For this review, take the finished solid that the model builds, in its own axes (mm). A direction names the side the tool comes from. Round coordinates to 2 decimals unless told otherwise and drop trailing zeros. Loops run counter-clockwise (first coordinate to the right, second up) from the corner with the lowest first, then second, coordinate; pieces in that order, holes last.
1) Take a section at C-C (y = 0). State the section outline as (x, z) points, then the cut area to 3 significant figures.
2) Tool access review of faces 1 (the flat face through (12, -17.828, -27)), 2 (the flat face through (12, -32.828, -19)), 3 (the cylindrical face through (12.325, -39.352, -60.393)): name each direction out of +Z, -Z, +X, -X, +Y, -Y from which nothing blocks a thin tool from reaching the whole face with its end or side.
3) Mouldability with a two-part tool opening along Z and no side actions: class faces 4 (the flat face through (0, 11.3, -26)), 5 (the cylindrical face through (12.32, -22.07, 24.3)), 6 (the flat face through (12.325, 18.802, -57.745)) as pulls with the +Z half, pulls with the -Z half, needs draft (parallel to the pull), parting line crosses it, or undercut.
4) Wall thickness on L1, parallel to Y at x = 11.5, z = -9.5; L2, parallel to Z at x = 7.5, y = 11.5; L3, parallel to Z at x = 7, y = 16: over which ranges is each line inside the solid? List them lowest first.
5) Insertion check: pin 1 (7.5 mm diameter, centred on x = 17, z = -40, fed in from -Y); pin 2 (10 mm diameter, centred on x = 17, y = 22.5, fed in from +Z); pin 3 (8 mm diameter, centred on x = 5, y = 3.5, fed in from +Z); pin 4 (10 mm diameter, centred on y = 5, z = -37, fed in from -X). Each pin has a flat end and moves straight along its axis. Give the tip position at first contact, or say it passes through.
6) Take a section at B-B (x = 18.5). State the section outline as (y, z) points, then the cut area to 3 significant figures.
7) Take a section at D-D (z = -32). State the section outline as (x, y) points.
8) Take a section at A-A (z = 6.5). State the section outline as (x, y) points.
```python
from build123d import *

# Parameters (mm, degrees)
F1_DEPTH = 25


# Not quite as in the source:
# - a feature names something its author has since deleted; it is built from what else it names


with BuildPart() as f1:
    # F0 (on Right) → F1 (new body)
    with BuildSketch(Plane.YZ):
        with BuildLine():
            Line((21.3200338185, 0), (17.8281293297, 0))
            ThreePointArc((17.8281293297, 0), (16.0680734174, -7.7239376), (11.135423556, -13.9228063846))
            Line((11.135423556, -13.9228063846), (11.135423556, -30.8818460833))
            ThreePointArc((11.135423556, -30.8818460833), (16.4953904054, -28.3828851715), (21.3200338185, -24.9628170138))
            Line((21.3200338185, -24.9628170138), (21.3200338185, 0))
        make_face()
        with BuildLine():
            ThreePointArc((-17.8281293297, 0), (0, 17.8281293297), (17.8281293297, 0))
            Line((17.8281293297, 0), (21.3200338185, 0))
            Line((21.3200338185, 0), (21.3200338185, -24.9628170138))
            ThreePointArc((21.3200338185, -24.9628170138), (29.8126055788, -13.7438940584), (32.8281293297, 0))
            ThreePointArc((32.8281293297, 0), (32.5773816899, 4.0497256101), (31.8289692891, 8.0375860357))
            Line((31.8289692891, 8.0375860357), (31.3856816717, 9.6241914615))
            ThreePointArc((31.3856816717, 9.6241914615), (28.3999929291, 16.4659186477), (23.9458348633, 22.4562478608))
            ThreePointArc((23.9458348633, 22.4562478608), (8.5005350475, 17.8111454186), (2.3973170077, 32.7404787144))
            ThreePointArc((2.3973170077, 32.7404787144), (-22.3493472221, 24.0456389815), (-32.8281293297, 0))
            Line((-32.8281293297, 0), (-17.8281293297, 0))
        make_face()
        with BuildLine():
            Line((-17.8281293297, -27.5652658229), (-17.8281293297, 0))
            Line((-17.8281293297, 0), (-32.8281293297, 0))
            ThreePointArc((-32.8281293297, 0), (-28.8353100436, -15.6911111771), (-17.8281293297, -27.5652658229))
        make_face()
        with BuildLine():
            Line((-17.8281293297, -49.2888468657), (-17.8281293297, -27.5652658229))
            ThreePointArc((-17.8281293297, -27.5652658229), (-28.8353100436, -15.6911111771), (-32.8281293297, 0))
            Line((-32.8281293297, 0), (-32.8281293297, -39.2883635356))
            ThreePointArc((-32.8281293297, -39.2883635356), (-23.2296585262, -41.1410511261), (-17.8281293297, -49.2888468657))
        make_face()
        with BuildLine():
            ThreePointArc((21.3200338185, -24.9628170138), (16.4953904054, -28.3828851715), (11.135423556, -30.8818460833))
            Line((11.135423556, -30.8818460833), (11.135423556, -91.2536308169))
            Line((11.135423556, -91.2536308169), (16.2277286872, -91.2536308169))
            Line((16.2277286872, -91.2536308169), (16.3531204545, -89.621300844))
            Line((16.3531204545, -89.621300844), (21.3200338185, -24.9628170138))
        make_face()
        with BuildLine():
            Line((-17.8281293297, -49.3592731655), (-17.8281293297, -49.2888468657))
            ThreePointArc((-17.8281293297, -49.2888468657), (-23.2296585262, -41.1410511261), (-32.8281293297, -39.2883635356))
            Line((-32.8281293297, -39.2883635356), (-32.8281293297, -49.3592731655))
            Line((-32.8281293297, -49.3592731655), (-17.8281293297, -49.3592731655))
        make_face()
        with BuildLine():
            ThreePointArc((24.9010812958, 32.8337324859), (13.6167044371, 40.6286479576), (2.3973170077, 32.7404787144))
            ThreePointArc((2.3973170077, 32.7404787144), (14.1397228999, 29.626918699), (23.9458348633, 22.4562478608))
            ThreePointArc((23.9458348633, 22.4562478608), (25.2235009878, 25.4290316666), (25.6599794461, 28.6351758987))
            ThreePointArc((25.6599794461, 28.6351758987), (25.6074521104, 29.7564349958), (25.4503302031, 30.867872709))
            Line((25.4503302031, 30.867872709), (24.9010812958, 32.8337324859))
        make_face()
        with BuildLine():
            ThreePointArc((23.9458348633, 22.4562478608), (14.1397228999, 29.626918699), (2.3973170077, 32.7404787144))
            ThreePointArc((2.3973170077, 32.7404787144), (8.5005350475, 17.8111454186), (23.9458348633, 22.4562478608))
        make_face()
        with BuildLine():
            Line((-32.8281293297, -49.3592731655), (-32.8281293297, -39.2883635356))
            ThreePointArc((-32.8281293297, -39.2883635356), (-39.0840214493, -60.6643501174), (-17.8281293297, -54.0118288841))
            Line((-17.8281293297, -54.0118288841), (-17.8281293297, -49.3592731655))
            Line((-17.8281293297, -49.3592731655), (-32.8281293297, -49.3592731655))
        make_face()
        Polygon((16.2277286872, -91.2536308169), (11.135423556, -91.2536308169), (13.3315734565, -94.4593122868), (17.8637079006, -94.4593122868), (19.3015802652, -93.3099836111), (17.6578841403, -91.2536308169), align=None)
        Polygon((17.6578841403, -91.2536308169), (16.3531204545, -89.621300844), (16.2277286872, -91.2536308169), align=None)
        with BuildLine():
            ThreePointArc((25.6599794461, 28.6351758987), (25.2235009878, 25.4290316666), (23.9458348633, 22.4562478608))
            ThreePointArc((23.9458348633, 22.4562478608), (28.3999929291, 16.4659186477), (31.3856816717, 9.6241914615))
            Line((31.3856816717, 9.6241914615), (25.4503302031, 30.867872709))
            ThreePointArc((25.4503302031, 30.867872709), (25.6074521104, 29.7564349958), (25.6599794461, 28.6351758987))
        make_face()
        with BuildLine():
            Line((31.3856816717, 9.6241914615), (31.8289692891, 8.0375860357))
            ThreePointArc((31.8289692891, 8.0375860357), (31.6172793456, 8.8336697962), (31.3856816717, 9.6241914615))
        make_face()
    extrude(amount=F1_DEPTH)


solid = f1.part
```
Response:
1. outline: (0, 17.83) - (25, 17.83) - (25, 32.83) - (0, 32.83) - close
1. area: 375 mm2
2. face 1: -Z, +X, -X
2. face 2: +Z, +X, -X, -Y
2. face 3: +X, -X
3. face 4: needs draft
3. face 5: pulls with the +Z half
3. face 6: undercut
4. L1: y = -32.83 to -17.83, 15.09 to 31.42
4. L2: z = -91.79 to -13.62, 13.62 to 40.43
4. L3: z = -94.46 to -7.86, 7.86 to 40.4
5. pin 1: stops at y = -40.09
5. pin 2: stops at z = 40
5. pin 3: stops at z = 38.92
5. pin 4: passes through
6. outline: (-32.83, -39.29) arc R12.63 ccw (long way) to (-17.83, -54.01) - (-17.83, 0) arc R17.83 cw (long way) to (11.14, -13.92) - (11.14, -91.25) - (13.33, -94.46) - (17.86, -94.46) - (19.3, -93.31) - (16.35, -89.62) - (21.32, -24.96) arc R32.83 ccw to (31.39, 9.62) - (24.9, 32.83) arc R11.99 ccw to (2.4, 32.74) arc R32.83 ccw to (-32.83, 0) - close
6. area: 3,470 mm2
7. outline: (0, -32.83) - (25, -32.83) - (25, -17.83) - (0, -17.83) - close; (0, 11.14) - (25, 11.14) - (25, 20.78) - (0, 20.78) - close
8. outline: (0, -32.18) - (25, -32.18) - (25, -16.6) - (0, -16.6) - close; (0, 16.6) - (25, 16.6) - (25, 32.18) - (0, 32.18) - close
